Part model, mm, in its own coordinate system. A direction names the side the tool comes from. Round coordinates to 2 decimals unless told otherwise and drop trailing zeros. Order: outer loops, then holes, each group sorted by start corner. A loop starts at its lowest first (then second) coordinate and runs counter-clockwise, first axis right, second up. Notation, with made-up numbers: M -9.75,31 L -0.75,31 A10 cw -0.75,35 Z; hole C 18.25,80 d6. An arc over 180 degrees is marked long. One line per question, with ' | ' between items.
from build123d import *

# Parameters (mm, degrees)
SKETCH2_W           = 63
SKETCH2_H           = 25
BOSS_EXTRUDE2_DEPTH = 20
SKETCH5_W           = 43
SKETCH5_H           = 25
CUT_EXTRUDE2_DEPTH  = 1
SKETCH6_W           = 10
SKETCH6_H           = 12
CUT_EXTRUDE3_DEPTH  = 10
CUT_EXTRUDE4_DEPTH  = 24
SKETCH8_W           = 43
SKETCH8_H           = 3
CUT_EXTRUDE5_DEPTH  = 8
SKETCH9_R           = 2
CUT_EXTRUDE6_DEPTH  = 4
SKETCH10_R          = 4.5
CUT_EXTRUDE7_DEPTH  = 19
SKETCH11_R          = 2
CUT_EXTRUDE8_DEPTH  = 19


with BuildPart() as part:
    # Sketch2 → Boss-Extrude2 (new body)
    with BuildSketch(Plane(origin=(0, 0, 0), x_dir=(1, 0, 0), z_dir=(0, 1, 0))):
        Rectangle(SKETCH2_W, SKETCH2_H)
    extrude(amount=BOSS_EXTRUDE2_DEPTH)

    # Sketch5 → Cut-Extrude2 (cut)
    with BuildSketch(Plane(origin=(0, 20, 0), x_dir=(1, 0, 0), z_dir=(0, 1, 0))):
        Rectangle(SKETCH5_W, SKETCH5_H)
    extrude(amount=-CUT_EXTRUDE2_DEPTH, mode=Mode.SUBTRACT)

    # Sketch6 → Cut-Extrude3 (cut)
    with BuildSketch(Plane(origin=(0, 19, 0), x_dir=(1, 0, 0), z_dir=(0, 1, 0))):
        with Locations((-16.5, 6.5)):
            Rectangle(SKETCH6_W, SKETCH6_H)
        with Locations((-16.5, -6.5)):
            Rectangle(SKETCH6_W, SKETCH6_H)
        with Locations((-5.5, -6.5)):
            Rectangle(SKETCH6_W, SKETCH6_H)
        with Locations((-5.5, 6.5)):
            Rectangle(SKETCH6_W, SKETCH6_H)
        with Locations((5.5, 6.5)):
            Rectangle(SKETCH6_W, SKETCH6_H)
        with Locations((5.5, -6.5)):
            Rectangle(SKETCH6_W, SKETCH6_H)
        with Locations((16.5, -6.5)):
            Rectangle(SKETCH6_W, SKETCH6_H)
        with Locations((16.5, 6.5)):
            Rectangle(SKETCH6_W, SKETCH6_H)
    extrude(amount=-CUT_EXTRUDE3_DEPTH, mode=Mode.SUBTRACT)

    # Sketch7 → Cut-Extrude4 (cut)
    with BuildSketch(Plane.XY.offset(12.5)):
        Polygon((-21.5, 9), (-11.5, 9), (-11.5, 8.5), (-12.5, 8.5), (-12.5, 7.5), (-20.5, 7.5), (-20.5, 8.5), (-21.5, 8.5), align=None)
        Polygon((-10.5, 9), (-0.5, 9), (-0.5, 8.5), (-1.5, 8.5), (-1.5, 7.5), (-9.5, 7.5), (-9.5, 8.5), (-10.5, 8.5), align=None)
        Polygon((0.5, 9), (10.5, 9), (10.5, 8.5), (9.5, 8.5), (9.5, 7.5), (1.5, 7.5), (1.5, 8.5), (0.5, 8.5), align=None)
        Polygon((11.5, 9), (21.5, 9), (21.5, 8.5), (20.5, 8.5), (20.5, 7.5), (12.5, 7.5), (12.5, 8.5), (11.5, 8.5), align=None)
    extrude(amount=-CUT_EXTRUDE4_DEPTH, mode=Mode.SUBTRACT)

    # Sketch8 → Cut-Extrude5 (cut)
    with BuildSketch(Plane.XZ):
        Rectangle(SKETCH8_W, SKETCH8_H)
    extrude(amount=-CUT_EXTRUDE5_DEPTH, mode=Mode.SUBTRACT)

    # Sketch9 → Cut-Extrude6 (cut)
    with BuildSketch(Plane(origin=(0, 7.5, 0), x_dir=(1, 0, 0), z_dir=(0, 1, 0))):
        with Locations(Location((-16.5, -7, 0), (0, 0, 270))):
            Circle(SKETCH9_R)
        with Locations(Location((-5.5, -7, 0), (0, 0, 270))):
            Circle(SKETCH9_R)
        with Locations(Location((5.5, -7, 0), (0, 0, 270))):
            Circle(SKETCH9_R)
        with Locations(Location((16.5, -7, 0), (0, 0, 270))):
            Circle(SKETCH9_R)
        with Locations(Location((16.5, 7, 0), (0, 0, 90))):
            Circle(SKETCH9_R)
        with Locations(Location((5.5, 7, 0), (0, 0, 90))):
            Circle(SKETCH9_R)
        with Locations(Location((-5.5, 7, 0), (0, 0, 90))):
            Circle(SKETCH9_R)
        with Locations(Location((-16.5, 7, 0), (0, 0, 90))):
            Circle(SKETCH9_R)
    extrude(amount=-CUT_EXTRUDE6_DEPTH, mode=Mode.SUBTRACT)

    # Sketch10 → Cut-Extrude7 (cut)
    with BuildSketch(Plane(origin=(0, 20, 0), x_dir=(1, 0, 0), z_dir=(0, 1, 0))):
        with Locations(Location((26.5, 0, 0), (0, 0, 270))):
            Circle(SKETCH10_R)
        with Locations(Location((-26.5, -0.5, 0), (0, 0, 270))):
            Circle(SKETCH10_R)
    extrude(amount=-CUT_EXTRUDE7_DEPTH, mode=Mode.SUBTRACT)

    # Sketch11 → Cut-Extrude8 (cut)
    with BuildSketch(Plane(origin=(0, 1, 0), x_dir=(1, 0, 0), z_dir=(0, 1, 0))):
        with Locations(Location((-26.5, -0.5, 0), (0, 0, 270))):
            Circle(SKETCH11_R)
        with Locations(Location((26.5, 0, 0), (0, 0, 270))):
            Circle(SKETCH11_R)
    extrude(amount=-CUT_EXTRUDE8_DEPTH, mode=Mode.SUBTRACT)


solid = part.part
1) Probe line 1 (X direction, y = 5.05, z = -7); line 2 (X direction, y = 12.5, z = 5.25); line 3 (Z direction, x = 21, y = 3). List the from-to ranges inside material, lowest first. Write a range as [from, to].
The answers:
line 1: x = [-31.5, -18.5], [-14.5, -7.5], [-3.5, 3.5], [7.5, 14.5], [18.5, 31.5] | line 2: x = [-31.5, -21.5], [-11.5, -10.5], [-0.5, 0.5], [10.5, 11.5], [21.5, 31.5] | line 3: z = [-12.5, -1.5], [1.5, 12.5]
2) Saw through at A-A (x = 5.5). List the corners of the cut face in (y, z), plus the area to 4 significant figures.
The answers:
outline: M 0,-12.5 L 9,-12.5 L 9,-11.5 L 7.5,-11.5 L 7.5,-9 L 3.5,-9 L 3.5,-5 L 7.5,-5 L 7.5,-1.5 L 0,-1.5 Z; M 0,1.5 L 7.5,1.5 L 7.5,5 L 3.5,5 L 3.5,9 L 7.5,9 L 7.5,12.5 L 0,12.5 Z; M 9,-0.5 L 19,-0.5 L 19,0.5 L 9,0.5 Z | area: 144.5 mm²
3) Which spindle directions (+Z, -Z, +X, -X, +Y, -Y) get a long thin tool onto all of the face, cutting with end or side? Do faces 5 (the face through (5, 14, -0.5)), 6 (the face through (22, 20, -3)), 7 (the face through (5, 3.5, -7)), 8 (the face through (16, 14, 0.5)). Say none if no direction does.
The answers:
face 5: -Z, +Y | face 6: +Z, -Z, +X, -X, +Y | face 7: +Y | face 8: +Z, +Y
4) Saw through at B-B (x = -26.5). List the corners of the cut face in (y, z).
The answers:
outline: M 0,-12.5 L 20,-12.5 L 20,-4 L 1,-4 L 1,-1.5 L 0,-1.5 Z; M 0,2.5 L 1,2.5 L 1,5 L 20,5 L 20,12.5 L 0,12.5 Z
5) Drop flat-ended pins along their axis: pin 1 (2 mm diameter, centred on x = -5.5, z = -6.5, fed in from +Y); pin 2 (1.2 mm diameter, centred on x = 5, y = 8.5, fed in from +Z); pin 3 (7.5 mm diameter, centred on x = -5, z = -1.5, fed in from +Y). Give the stop position or say it passes through.
The answers:
pin 1: stops at y = 3.5 | pin 2: stops at z = 0.5 | pin 3: stops at y = 19
6) Saw through at C-C (y = 6). Give the number of separate pieces and of enclosed holes in the cut face, plus the area to 3 significant figures.
The answers:
separate pieces: 1 | enclosed holes: 11 | area: 1,220 mm²
7) Two-plate mould, pull along X, no slides. Class faces 1 (the face through (-28.452, 0.507, 0.066)), 2 (the face through (31.5, 10, 0)), 3 (the face through (0, 8, -12.5)), 4 (the face through (-6, 3.5, -7)): released by +X, released by -X, zero draft, split by the parting line, or undercut.
The answers:
face 1: undercut | face 2: released by +X | face 3: zero draft | face 4: undercut
